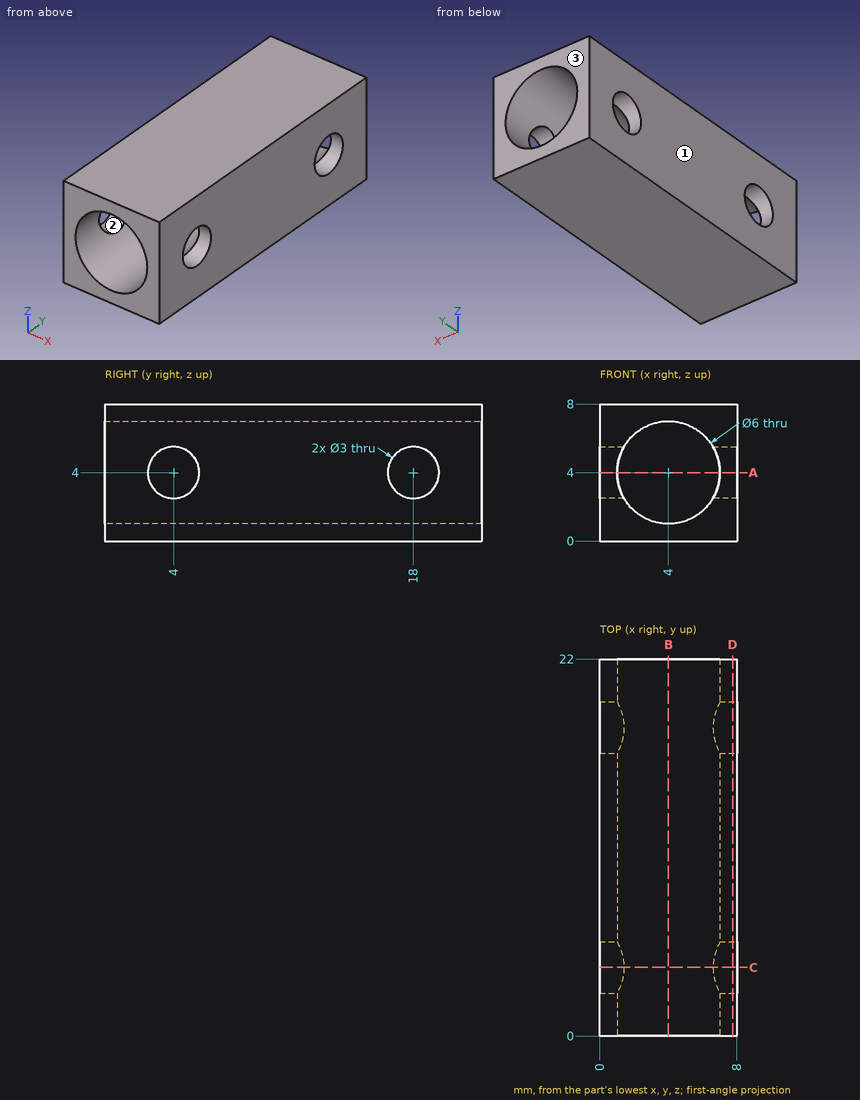
Check sheet for the drawn part. Datum: minimum x, y, z corner. Units: mm. Round coordinates to 2 decimals unless told otherwise and drop trailing zeros. Loops run counter-clockwise (first coordinate to the right, second up) from the corner with the lowest first, then second, coordinate; pieces in that order, holes last. Notation, with made-up numbers: M 22.5,62.5 L 29.5,62.5 A14 cw 29.5,79.5 Z; hole C -3,-40 d2. An arc over 180 degrees is marked long. One line per question, with ' | ' between items. Start each with the question number.
Item 1: Section check C-C (y = 4). Record the boundary of the cut face in (x, z), and give its area (3 significant figures).
Item 2: Section check B-B (x = 4). Record the boundary of the cut face in (y, z), and give its area (3 significant figures).
Item 3: Scan lines: probe 1 along Y at (x, z) = (0.3, 4); probe 2 along X at (y, z) = (6.25, 4); probe 3 along Z at (x, y) = (5.5, 5.25). Record each from-to range of solid material in increasing order.
Item 4: Release check for a two-part mould opening along Y. For the marked faces 1, 2 and 3 record: released by +Y, released by -Y, zero draft, split by the parting line, or undercut.
Item 5: Section check A-A (z = 4). Record the boundary of the cut face in (x, y), and give its area (3 significant figures).
Item 6: Section check D-D (x = 7.75). Record the boundary of the cut face in (y, z).
Worked out:
1) outline: M 0,0 L 8,0 L 8,2.5 L 6.6,2.5 A3 cw 1.4,2.5 L 0,2.5 Z; M 0,5.5 L 1.4,5.5 A3 cw 6.6,5.5 L 8,5.5 L 8,8 L 0,8 Z | area: 28.9 mm^2
2) outline: M 0,0 L 22,0 L 22,1 L 0,1 Z; M 0,7 L 22,7 L 22,8 L 0,8 Z | area: 44.0 mm^2
3) probe 1: 0 to 2.5, 5.5 to 16.5, 19.5 to 22 | probe 2: 0 to 1, 7 to 8 | probe 3: 0 to 1.4, 6.6 to 8
4) face 1: zero draft | face 2: undercut | face 3: released by +Y
5) outline: M 0,0 L 1,0 L 1,2.5 L 0,2.5 Z; M 0,5.5 L 1,5.5 L 1,16.5 L 0,16.5 Z; M 0,19.5 L 1,19.5 L 1,22 L 0,22 Z; M 7,0 L 8,0 L 8,2.5 L 7,2.5 Z; M 7,5.5 L 8,5.5 L 8,16.5 L 7,16.5 Z; M 7,19.5 L 8,19.5 L 8,22 L 7,22 Z | area: 32.0 mm^2
6) outline: M 0,0 L 22,0 L 22,8 L 0,8 Z; hole C 4,4 d3; hole C 18,4 d3
